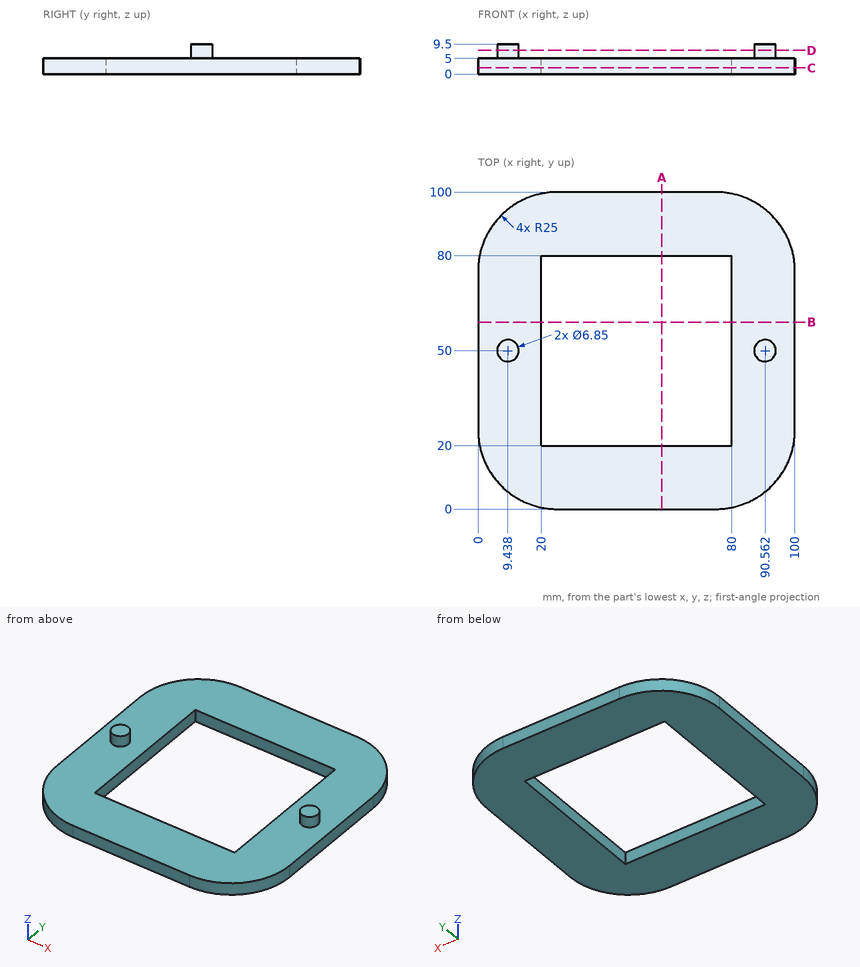
Drawing for the job (mm, zero at the part's lowest x, y, z). Coordinates: 2 decimals unless noted, no trailing zeros. Order: outer loops, then holes, each group sorted by start corner. A loop starts at its lowest first (then second) coordinate and runs counter-clockwise, first axis right, second up. Notation, with made-up numbers: (19.25, 32.5) -> (57.25, 32.5) arc R15 ccw to (57.25, 46.5) -> close; hole circle Ø7 at (57.25, 71.5). An arc over 180 degrees is marked (long way). Return JSON: item names as keys, results as strings.
Item 1: Slice it at C-C (z = 2). Write the cut outline in (x, y).
Model answer:
{"outline": "(0, 25) arc R25 ccw to (25, 0) -> (75, 0) arc R25 ccw to (100, 25) -> (100, 75) arc R25 ccw to (75, 100) -> (25, 100) arc R25 ccw to (0, 75) -> close; hole (20, 20) -> (80, 20) -> (80, 80) -> (20, 80) -> close"}
Item 2: Wall check: line 1 along X through (y, z) = (63.5, 3.5); line 2 along Z through (x, y) = (67.5, 86.5). Give the ranges that are in metal, low to high. Write a range as from..to.
Model answer:
{"line 1": "x = 0..20, 80..100", "line 2": "z = 0..5"}
Item 3: Slice it at D-D (z = 7.5). Write the cut outline in (x, y) (3 decimals), then the cut area to 3 significant figures.
Model answer:
{"outline": "circle Ø6.85 at (9.438, 50); circle Ø6.85 at (90.562, 50)", "area": "73.7 mm²"}
Item 4: Pin check, flat tip, straight feed: P1, Ø5, axis at y = 85.5, z = 6.5, coming from the +X side. Stop position of the tip, or through.
Model answer:
{"P1": "stops at x = 98.51"}
Item 5: Slice it at A-A (x = 58). Write the cut outline in (y, z), then the cut area to 3 significant figures.
Model answer:
{"outline": "(0, 0) -> (20, 0) -> (20, 5) -> (0, 5) -> close; (80, 0) -> (100, 0) -> (100, 5) -> (80, 5) -> close", "area": "200 mm²"}
